Autodesk Inventor part; units mm, degrees
ref_plane "YZ Plane" through (0, 0, 0) normal (1, 0, 0) x (0, 1, 0)
ref_plane "XZ Plane" through (0, 0, 0) normal (0, 1, 0) x (-1, 0, 0)
ref_plane "XY Plane" through (0, 0, 0) normal (0, 0, 1) x (1, 0, 0)
sketch "Sketch1" plane through (0, 0, 0) normal (0, 0, 1) x (1, 0, 0)
  line L0 (0, 0) -> (30, 0)
  line L1 (30, 0) -> (30, 15.6)
  line L2 (30, 15.6) -> (0, 15.6)
  line L3 (0, 15.6) -> (0, 0)
  dimension "d0" = 30
  dimension "d1" = 15.6
extrude "Extrusion1" add sketch "Sketch1" along normal blind 15.6
sketch "Sketch2" plane through (30, 0, 0) normal (1, 0, 0) x (0, 0, -1)
  line L0 (0, 0) -> (0, 15.6)
  line L1 (0, 15.6) -> (-15.6, 15.6)
  line L2 (-15.6, 0) -> (-15.6, 15.6)
  line L3 (0, 0) -> (-15.6, 0)
  circle A0 centre (-7.8, 7.8) radius 2.9
  dimension "d4" = 5.8
extrude "Extrusion2" add sketch "Sketch2" along normal blind 17 contours A0
sketch "Sketch3" plane through (0, 0, 0) normal (-1, 0, 0) x (0, 0, 1)
  circle A0 centre (7.8, 7.8) radius 2.9
  circle A1 centre (7.8, 7.8) radius 1.425
  point P0 (0, 0)
  dimension "d7" = 2.85
extrude "Extrusion3" add sketch "Sketch3" along normal blind 15 contours A1
fillet "Fillet1" radius 1 1 edges at (-15, 7.8, 6.375)
sketch "Sketch4" plane through (0, 15.6, 0) normal (0, 1, 0) x (1, 0, 0)
  circle A0 centre (8, -7.8101) radius 1.4
  circle A1 centre (22, -7.8101) radius 1.4
  line L0 (30, 0) -> (30, -15.6)
  line L1 (0, 0) -> (0, -15.6)
  dimension "d11" = 2.8
  dimension "d12" = 2.8
  dimension "d13" = 8
  dimension "d14" = 8
extrude "Extrusion4" cut sketch "Sketch4" against normal blind 5
properties part number "00_JF-0530B-solenoid"
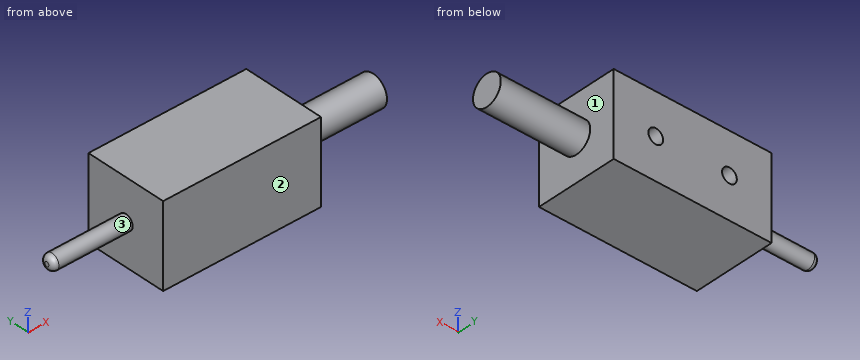
Input: part model. Units: mm. Frame: model coordinates. Face numbers are marked on the shaded views. A direction names the side the tool comes from. Round coordinates to 2 decimals unless told otherwise and drop trailing zeros. Order: outer loops, then holes, each group sorted by start corner. A loop starts at its lowest first (then second) coordinate and runs counter-clockwise, first axis right, second up.
1. Pin query (flat end, axial travel): P1, Ø2, axis at y = 12, z = 6.5, coming from the -X side; P2, Ø1.5, axis at y = 11.5, z = 4, coming from the +X side; P3, Ø6, axis at x = 38, z = 6, coming from the +Y side. Return the tip coordinate at first contact, or that it passes through.
The answers:
P1: stops at x = 0
P2: stops at x = 30
P3: stops at y = 10.7
2. Cut plane A-A, the plane x = 22. Output: boundary loops of the cut face in (y, z).
The answers:
outline: (0, 0) - (15.6, 0) - (15.6, 6.41) - (10.6, 6.41) - (10.6, 9.21) - (15.6, 9.21) - (15.6, 15.6) - (0, 15.6) - close
3. Set-up query: the marked faces 1, 2 and 3. Return all of +Z, -Z, +X, -X, +Y, -Y with unobstructed straight access to the full face (end or side cutting, diameter ignored); none if empty.
The answers:
face 1: +X
face 2: +Z, -Z, +X, -X, -Y
face 3: -X
4. Cut plane B-B, the plane y = 12.5. Output: boundary loops of the cut face in (x, z), then the cut area to 3 significant figures.
The answers:
outline: (0, 0) - (30, 0) - (30, 15.6) - (0, 15.6) - close; hole circle Ø2.8 at (8, 7.81); hole circle Ø2.8 at (22, 7.81)
area: 456 mm2
5. Material intervals for line 1 (Z direction, x = 8, y = 12.15); line 2 (X direction, y = 9.25, z = 15); line 3 (X direction, y = 12, z = 9), sorted ascending.
The answers:
line 1: z = 0 to 6.41, 9.21 to 15.6
line 2: x = 0 to 30
line 3: x = 0 to 7.26, 8.74 to 21.26, 22.74 to 30
6. Cut plane C-C, the plane z = 4. Output: boundary loops of the cut face in (x, y), then the cut area to 3 significant figures.
The answers:
outline: (0, 0) - (30, 0) - (30, 15.6) - (0, 15.6) - close
area: 468 mm2
